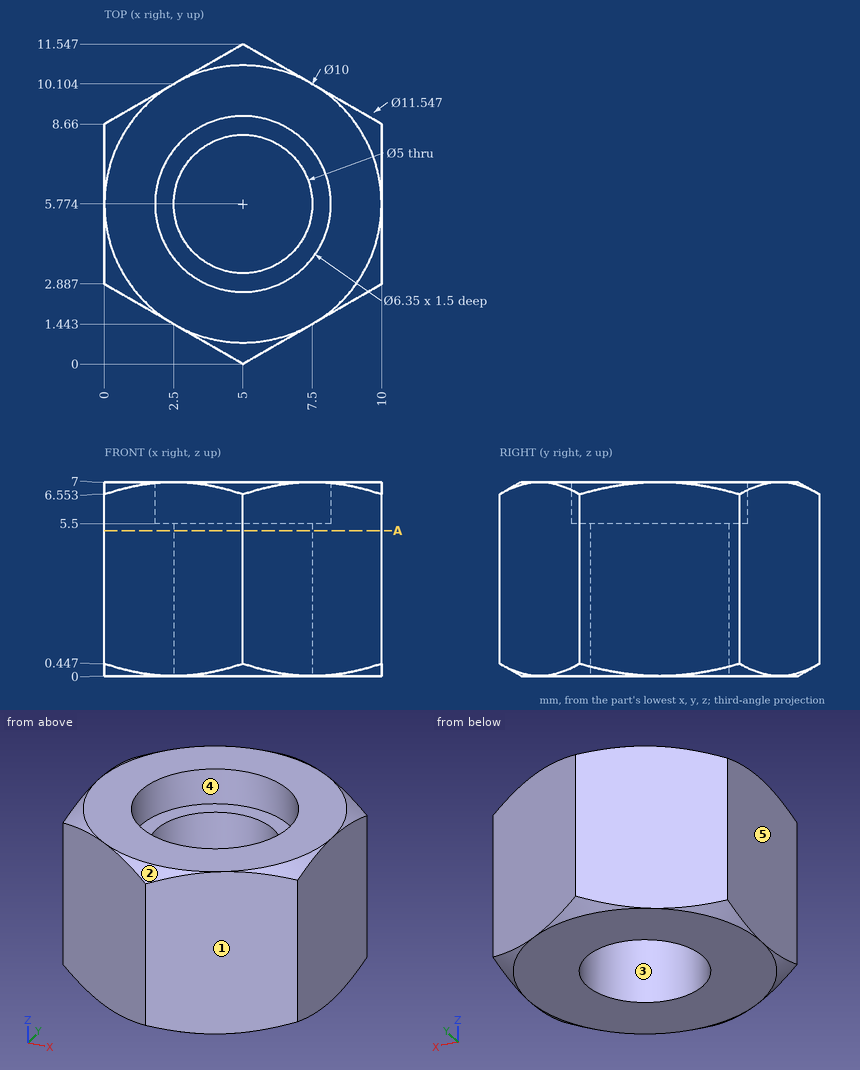
Study the drawing (mm; zero at the part's minimum x, y, z) and answer. A direction names the side the tool comes from. Give positions to 0.01 mm unless a question says otherwise; leave off trailing zeros. Order: outer loops, then holes, each group sorted by start corner. A loop starts at its lowest first (then second) coordinate and runs counter-clockwise, first axis right, second up. Notation, with made-up numbers: (79, 2) - (124, 2) arc R12 ccw to (124, 11) - close; hole circle Ø6 at (-14, 64). An arc over 180 degrees is marked (long way). Answer in a Markdown table with one row per item. Add a question column.
Q1. Which of the six approach directions +Z, -Z, +X, -X, +Y, -Y give full straight-line access (tool end or side, diameter ignored) to the marked faces 4 and 5?
Q2. Find the intervals of material crossed by line 1 along X through (y, z) = (6, 4); line 2 along Z through (x, y) = (4, 3.25); line 3 along X through (y, z) = (6, 6.25), in increasing order. Write a range as [from, to].
Q3. For a pull along X with two mould halves and no side action, classify the marked faces 1, 2 and 3 as released by +X, released by -X, zero draft, split by the parting line, or undercut.
Q4. The part is cut by section A-A (z = 5.25). Determine the outline of the cut face in (x, y).
Q5. Given P1, Ø1.5, axis at x = 3.5, z = 6, coming from the +Y side (1 decimal), flat-ended and moving along its own axis, determine where the tip first touches the part or whether it passes through.
Determined:
| question | item | result |
|---|---|---|
| 1 | face 4 | +Z |
| 1 | face 5 | +Z, -Z, -X, +Y, -Y |
| 2 | line 1 | x = [0, 2.51], [7.49, 10] |
| 2 | line 2 | z = [0, 5.5] |
| 2 | line 3 | x = [0, 1.83], [8.17, 10] |
| 3 | face 1 | released by +X |
| 3 | face 2 | split by the parting line |
| 3 | face 3 | undercut |
| 4 | outline | (0, 2.89) - (5, 0) - (10, 2.89) - (10, 8.66) - (5, 11.55) - (0, 8.66) - close; hole circle Ø5 at (5, 5.77) |
| 5 | P1 | stops at y = 11.1 |
